from build123d import *

# Parameters (mm, degrees)
SKETCH1_W             = 5.683554567
SKETCH1_H             = 108.574669318
BOSS_EXTRUDE2_DEPTH   = 76.2
SKETCH1_W_2           = 5.307190744
BOSS_EXTRUDE2_2_DEPTH = 76.2
SKETCH1_5_W           = 116.519157318
SKETCH1_5_H           = 108.574669318
SKETCH1_5_R           = 1.5
SKETCH1_5_R_2         = 1.8
SKETCH1_5_R_3         = 0.875
SKETCH1_5_R_4         = 8.6768437
SKETCH1_5_W_2         = 5.683554567
SKETCH1_5_W_3         = 5.307190744
BOSS_EXTRUDE3_DEPTH   = 5


with BuildPart() as part:
    # Sketch1 → Boss-Extrude2 (new body)
    with BuildSketch(Plane(origin=(0, 0, 0), x_dir=(1, 0, 0), z_dir=(0, 1, 0))):
        with Locations((-61.101355943, 0)):
            Rectangle(SKETCH1_W, SKETCH1_H)
    extrude(amount=BOSS_EXTRUDE2_DEPTH)



with BuildPart() as body_2:
    # Sketch1 → Boss-Extrude2 2 (new body)
    with BuildSketch(Plane(origin=(0, 0, 0), x_dir=(1, 0, 0), z_dir=(0, 1, 0))):
        with Locations((60.913174031, 0)):
            Rectangle(SKETCH1_W_2, SKETCH1_H)
    extrude(amount=BOSS_EXTRUDE2_2_DEPTH)


with BuildPart() as part_1:
    add(part.part)

    add(body_2.part)  # Boss-Extrude3 merges body 2
    # Sketch1_5 → Boss-Extrude3 (add)
    # profile 1 of 3: a face of its own
    with BuildSketch(Plane(origin=(0, 0, 0), x_dir=(1, 0, 0), z_dir=(0, 1, 0))):
        Rectangle(SKETCH1_5_W, SKETCH1_5_H)
        with Locations(Location((-15.686506038, -16.834299163, 0), (0, 0, 270))):
            Circle(SKETCH1_5_R, mode=Mode.SUBTRACT)
        with Locations(Location((-15, 0, 0), (0, 0, 270))):
            Circle(SKETCH1_5_R_2, mode=Mode.SUBTRACT)
        with Locations(Location((0, -15, 0), (0, 0, 270))):
            Circle(SKETCH1_5_R_2, mode=Mode.SUBTRACT)
        with Locations(Location((16.834299163, -15.686506038, 0), (0, 0, 270))):
            Circle(SKETCH1_5_R, mode=Mode.SUBTRACT)
        with Locations(Location((11.328100331, -11.608727014, 0), (0, 0, 270))):
            Circle(SKETCH1_5_R_3, mode=Mode.SUBTRACT)
        with Locations(Location((0, 0, 0), (0, 0, 270))):
            Circle(SKETCH1_5_R_4, mode=Mode.SUBTRACT)
        with Locations(Location((-11.328100331, 11.608727014, 0), (0, 0, 270))):
            Circle(SKETCH1_5_R_3, mode=Mode.SUBTRACT)
        with Locations(Location((-16.834299163, 15.686506038, 0), (0, 0, 270))):
            Circle(SKETCH1_5_R, mode=Mode.SUBTRACT)
        with Locations(Location((15, 0, 0), (0, 0, 270))):
            Circle(SKETCH1_5_R_2, mode=Mode.SUBTRACT)
        with Locations(Location((0, 15, 0), (0, 0, 270))):
            Circle(SKETCH1_5_R_2, mode=Mode.SUBTRACT)
        with Locations(Location((15.686506038, 16.834299163, 0), (0, 0, 270))):
            Circle(SKETCH1_5_R, mode=Mode.SUBTRACT)
    # profile 2 of 3: a face of its own
    with BuildSketch(Plane(origin=(0, 0, 0), x_dir=(1, 0, 0), z_dir=(0, 1, 0))):
        with Locations((-61.101355943, 0)):
            Rectangle(SKETCH1_5_W_2, SKETCH1_5_H)
    # profile 3 of 3: a face of its own
    with BuildSketch(Plane(origin=(0, 0, 0), x_dir=(1, 0, 0), z_dir=(0, 1, 0))):
        with Locations((60.913174031, 0)):
            Rectangle(SKETCH1_5_W_3, SKETCH1_5_H)
    extrude(amount=BOSS_EXTRUDE3_DEPTH)


solid = part_1.part
CAD build for the part. Positions are in the model's coordinates, mm. A direction names the side the tool comes from. Round coordinates to 2 decimals unless told otherwise and drop trailing zeros. Loops run counter-clockwise (first coordinate to the right, second up) from the corner with the lowest first, then second, coordinate; pieces in that order, holes last.
(1) Two-plate mould, pull along X, no slides. Class faces 3 (the flat face through (58.26, 40, 1)), 4 (the flat face through (63.567, 38, 1)), 5 (the flat face through (-58.26, 40, 1)), 6 (the flat face through (-63.943, 38, 1)): +X half, -X half, draft (parallel to the pull), parting line (faces both ways), or undercut.
(2) Cut at C-C (z = 0). Give the cut face in (x, y).
(3) Cut at B-B (x = 0). Give the cut face in (y, z).
(4) Wall check: line 1 along X through (y, z) = (3.25, 0); line 2 along X through (y, z) = (9, 8.5); line 3 along Y through (x, z) = (-45, 8). Give the ranges that are in metal, low to high.
(5) Drop flat-ended pins along their axis: pin 1 (1.1 mm diameter, centred on x = 11.33, z = 11.61, fed in from +Y); pin 2 (3.5 mm diameter, centred on x = -16.83, z = -15.69, fed in from +Y). Give the stop position or say it passes through.
(6) Which spindle directions (+Z, -Z, +X, -X, +Y, -Y) get a long thin tool onto all of the face, cutting with end or side? Do faces 1 (the flat face through (-1, 5, -13)), 2 (the cylindrical face through (16.785, 2.465, -0.234)). Say none if no direction does.
(7) Cut at A-A (y = 21). Give the cut face in (x, z).
(8) Cut at D-D (z = 32.5). Give the cut face in (x, y), plus the area to 3 significant figures.
Findings below:
1. face 3: undercut
1. face 4: +X half
1. face 5: undercut
1. face 6: -X half
2. outline: (-63.94, 0) - (-16.8, 0) - (-16.8, 5) - (-58.26, 5) - (-58.26, 76.2) - (-63.94, 76.2) - close; (-13.2, 0) - (-8.68, 0) - (-8.68, 5) - (-13.2, 5) - close; (8.68, 0) - (13.2, 0) - (13.2, 5) - (8.68, 5) - close; (16.8, 0) - (63.57, 0) - (63.57, 76.2) - (58.26, 76.2) - (58.26, 5) - (16.8, 5) - close
3. outline: (0, -54.29) - (5, -54.29) - (5, -16.8) - (0, -16.8) - close; (0, -13.2) - (5, -13.2) - (5, -8.68) - (0, -8.68) - close; (0, 8.68) - (5, 8.68) - (5, 13.2) - (0, 13.2) - close; (0, 16.8) - (5, 16.8) - (5, 54.29) - (0, 54.29) - close
4. line 1: x = -63.94 to -16.8, -13.2 to -8.68, 8.68 to 13.2, 16.8 to 63.57
4. line 2: x = -63.94 to -58.26, 58.26 to 63.57
4. line 3: y = 0 to 5
5. pin 1: passes through
5. pin 2: stops at y = 5
6. face 1: +Z, -Z, +Y
6. face 2: +Y, -Y
7. outline: (-63.94, -54.29) - (-58.26, -54.29) - (-58.26, 54.29) - (-63.94, 54.29) - close; (58.26, -54.29) - (63.57, -54.29) - (63.57, 54.29) - (58.26, 54.29) - close
8. outline: (-63.94, 0) - (63.57, 0) - (63.57, 76.2) - (58.26, 76.2) - (58.26, 5) - (-58.26, 5) - (-58.26, 76.2) - (-63.94, 76.2) - close
8. area: 1,420 mm2
